Verification items for the finished model (mm, model axes). A direction names the side the tool comes from. Round coordinates to 2 decimals unless told otherwise and drop trailing zeros. Order: outer loops, then holes, each group sorted by start corner. A loop starts at its lowest first (then second) coordinate and runs counter-clockwise, first axis right, second up. Notation, with made-up numbers: M -20,50 L 35,50 A24 cw 35,68 Z; hole C -21,61 d3. An arc over 180 degrees is marked long. Use CSV: the item, a comma, the result in double quotes. Start each with the question number.
Q1. Mould release check, pull along X, two halves, no side actions. Record for faces 3 (the face through (-0.867, -3.905, 2.979)), 4 (the face through (0, 0, 4.5)), 5 (the face through (-4, -4, 0.25)): +X half, -X half, draft (parallel to the pull), parting line (faces both ways), or undercut.
Q2. Gauge pin test, flat ends, axial feed: pin 1 Ø1.5 at (y, z) = (4, 1) entering from +X; pin 2 Ø2 at (x, z) = (-2.5, 2) entering from -Y; pin 3 Ø1.5 at (x, z) = (0, 2.5) entering from +Y. Record the tip position at first contact, or that the pin passes through.
Q3. Sectioned sample at A-A (z = 2.3). Enter the section's corners in (x, y).
Q4. Scan lines: line 1 (Z direction, x = 2.5, y = 3.5); line 2 (Z direction, x = 8, y = 3.75); line 3 (Y direction, x = 1.5, z = 2.25). Record each from-to range of solid material in increasing order.
Q5. Set-up check for faces 1 (the face through (4, -2, 1.5)), 2 (the face through (-2, -6, 0)): record each of +Z, -Z, +X, -X, +Y, -Y from which the full face is reachable in a straight line by a thin tool's end or side.
```python
from build123d import *

# Parameters (mm, degrees)
F0_R     = 9
F1_DEPTH = 1.5
F2_R     = 4
F3_DEPTH = 3
F5_R     = 6
F6_DEPTH = 0.25


# Not quite as in the source:
# - a fillet or chamfer that OpenCascade refuses, or shapes differently, is made with other operations: its cross-section is extruded or revolved along the edge and cut away or added


with BuildPart() as f1:
    # F0 (on Top) → F1 (new body)
    with BuildSketch(Plane.XY):
        Circle(F0_R)
    extrude(amount=F1_DEPTH)

    # F2 (on face) → F3 (join)
    with BuildSketch(Plane.XY.offset(1.5)):
        Circle(F2_R)
    extrude(amount=F3_DEPTH)

    # F4: fillet of radius 2 on 1 edges, made by hand

    # F4_s1 → F4_t2 (revolve, cut)
    with BuildSketch(Plane.XZ):
        with BuildLine():
            ThreePointArc((9, 1.5), (8.2882531983, 0.4188611699), (7.0635083269, 0))
            Line((7.0635083269, 0), (9, 0))
            Line((9, 0), (9, 1.5))
        make_face()
    revolve(axis=Axis((0, 0, 0), (0, 0, 1)), mode=Mode.SUBTRACT)

    # F5 (on face) → F6 (cut)
    with BuildSketch(Plane(origin=(0, 0, 0), x_dir=(1, 0, 0), z_dir=(0, 0, -1))):
        Circle(F5_R)
        with BuildLine():
            ThreePointArc((0, 5), (3.5355339059, 3.5355339059), (5, 0))
            ThreePointArc((5, 0), (3.5355339059, -3.5355339059), (0, -5))
            ThreePointArc((0, -5), (-3.5355339059, -3.5355339059), (-5, 0))
            ThreePointArc((-5, 0), (-3.5355339059, 3.5355339059), (0, 5))
        make_face(mode=Mode.SUBTRACT)
    extrude(amount=-F6_DEPTH, mode=Mode.SUBTRACT)


solid = f1.part
```
Verdict:
1,face 3,"parting line"
1,face 4,"draft"
1,face 5,"undercut"
2,pin 1,"stops at x = 8.32"
2,pin 2,"stops at y = -8.85"
2,pin 3,"stops at y = 4"
3,outline,"C 0,0 d8"
4,line 1,"z = 0 to 1.5"
4,line 2,"z = 1.07 to 1.5"
4,line 3,"y = -3.71 to 3.71"
5,face 1,"+Z"
5,face 2,"-Z, +X, -X, +Y, -Y"
